The listing builds one solid part. Answer for the finished solid, in the listing's coordinates (mm). Face numbers are marked on the shaded views. A direction names the side the tool comes from. Round coordinates to 2 decimals unless told otherwise and drop trailing zeros. Loops run counter-clockwise (first coordinate to the right, second up) from the corner with the lowest first, then second, coordinate; pieces in that order, holes last. Notation, with made-up numbers: (-34, 59.5) -> (-11, 59.5) arc R7 ccw to (-11, 69.5) -> close; hole circle Ø10 at (58, -13). An arc over 180 degrees is marked (long way). Use a Markdown table: item, result. Add a question column.
Q1. For a pull along X with two mould halves and no side action, classify the marked faces 1, 2 and 3 as released by +X, released by -X, zero draft, split by the parting line, or undercut.
Q2. Section D-D on x = -76.5 is taken. Give the vertices of the cut face in (y, z).
Q3. Which of the six approach directions +Z, -Z, +X, -X, +Y, -Y give full straight-line access (tool end or side, diameter ignored) to the marked faces 4 and 5?
Q4. Consider line 1 (Y direction, x = -97, z = 180); line 2 (X direction, y = 27.5, z = 146.5); line 3 (X direction, y = 5, z = 2). Determine where each line is inside the solid, lowest interval first.
Q5. Section A-A on x = -10.5 is taken. Give the vertices of the cut face in (y, z), then the cut area to 3 significant figures.
Q6. Given pin 1 Ø2 at (x, y) = (-96, 72.5) entering from +Z; pin 2 Ø1.5 at (x, z) = (52, 31) entering from +Y; pin 3 Ø9.5 at (x, z) = (-2, 89.5) entering from +Y; pin 4 Ø2.5 at (x, z) = (96, 98) entering from +Y, each flat-ended and moving along its own axis, determine where each tip first touches the part or whether it passes through.
Q7. Section C-C on y = 34 is taken. Give the vertices of the cut face in (x, z).
from build123d import *

# Parameters (mm, degrees)
BOSS_EXTRUDE1_DEPTH = 225
BOSS_EXTRUDE2_DEPTH = 10
SKETCH6_W           = 210
SKETCH6_H           = 200
BOSS_EXTRUDE3_DEPTH = 15
SKETCH5_R           = 2.1
CUT_EXTRUDE1_DEPTH  = 6
SKETCH10_W          = 210
SKETCH10_H          = 200
BOSS_EXTRUDE4_DEPTH = 40
SKETCH11_R          = 4.75
BOSS_EXTRUDE5_DEPTH = 5
BOSS_EXTRUDE5_TAPER = 5
SKETCH13_W          = 185
SKETCH13_H          = 10
BOSS_EXTRUDE6_DEPTH = 47.5
SKETCH14_W          = 185
SKETCH14_H          = 10
BOSS_EXTRUDE7_DEPTH = 47.5
SKETCH7_W           = 21
SKETCH7_H           = 10.25
CUT_EXTRUDE2_DEPTH  = 15
SKETCH15_R          = 2.1
CUT_EXTRUDE4_DEPTH  = 4.5
CUT_EXTRUDE5_DEPTH  = 185
SKETCH17_W          = 210
SKETCH17_H          = 40
BOSS_EXTRUDE8_DEPTH = 10


with BuildPart() as part:
    # Sketch2 → Boss-Extrude1 (new body)
    with BuildSketch(Plane(origin=(0, 0, 0), x_dir=(1, 0, 0), z_dir=(0, 1, 0))):
        Polygon((-90, 0), (90, 0), (90, -185), (105, -185), (105, 15), (-105, 15), (-105, -185), (-90, -185), align=None)
    extrude(amount=BOSS_EXTRUDE1_DEPTH)

    # Sketch3 → Boss-Extrude2 (add)
    with BuildSketch(Plane(origin=(0, 10, 0), x_dir=(1, 0, 0), z_dir=(0, 1, 0))):
        Polygon((-90, -185), (-22.5, -185), (-22.5, -10), (22.5, -10), (22.5, -185), (90, -185), (90, 0), (-90, 0), align=None)
    extrude(amount=BOSS_EXTRUDE2_DEPTH)

    # Sketch6 → Boss-Extrude3 (add)
    with BuildSketch(Plane.XZ):
        with Locations((0, 85)):
            Rectangle(SKETCH6_W, SKETCH6_H)
    extrude(amount=BOSS_EXTRUDE3_DEPTH)

    # Sketch5 → Cut-Extrude1 (cut)
    with BuildSketch(Plane.XY.offset(185)):
        with Locations((-97.5, 217.5)):
            Circle(SKETCH5_R)
        with Locations((97.5, 217.5)):
            Circle(SKETCH5_R)
        with Locations((-97.5, -7.5)):
            Circle(SKETCH5_R)
        with Locations((97.5, -7.5)):
            Circle(SKETCH5_R)
    extrude(amount=-CUT_EXTRUDE1_DEPTH, mode=Mode.SUBTRACT)

    # Sketch10 → Boss-Extrude4 (add)
    with BuildSketch(Plane.XZ.offset(15)):
        with Locations((0, 85)):
            Rectangle(SKETCH10_W, SKETCH10_H)
    extrude(amount=BOSS_EXTRUDE4_DEPTH)

    # Sketch11 → Boss-Extrude5 (add)
    with BuildSketch(Plane(origin=(0, 0, 0), x_dir=(1, 0, 0), z_dir=(0, 1, 0))):
        with Locations((0, -90)):
            Circle(SKETCH11_R)
    extrude(amount=BOSS_EXTRUDE5_DEPTH, taper=BOSS_EXTRUDE5_TAPER)

    # Sketch13 → Boss-Extrude6 (add)
    with BuildSketch(Plane.ZY.offset(-90)):
        with Locations((92.5, 5)):
            Rectangle(SKETCH13_W, SKETCH13_H)
    extrude(amount=BOSS_EXTRUDE6_DEPTH)

    # Sketch14 → Boss-Extrude7 (add)
    with BuildSketch(Plane(origin=(-90, 0, 0), x_dir=(0, 0, -1), z_dir=(1, 0, 0))):
        with Locations((-92.5, 5)):
            Rectangle(SKETCH14_W, SKETCH14_H)
    extrude(amount=BOSS_EXTRUDE7_DEPTH)

    # Sketch7 → Cut-Extrude2 (cut)
    with BuildSketch(Plane(origin=(0, 0, -15), x_dir=(-1, 0, 0), z_dir=(0, 0, -1))):
        with Locations((-32, 5.125)):
            Rectangle(SKETCH7_W, SKETCH7_H)
    extrude(amount=-CUT_EXTRUDE2_DEPTH, mode=Mode.SUBTRACT)

    # Sketch15 → Cut-Extrude4 (cut)
    with BuildSketch(Plane(origin=(0, 225, 0), x_dir=(1, 0, 0), z_dir=(0, 1, 0))):
        with Locations((0, 7.5)):
            Circle(SKETCH15_R)
        with Locations((-97.5, -90)):
            Circle(SKETCH15_R)
        with Locations((97.5, -90)):
            Circle(SKETCH15_R)
    extrude(amount=-CUT_EXTRUDE4_DEPTH, mode=Mode.SUBTRACT)

    # Split1
    split(bisect_by=Plane.ZX.offset(75), keep=Keep.BOTTOM)

    # Sketch16 → Cut-Extrude5 (cut)
    with BuildSketch(Plane.XY.offset(185)):
        Polygon((-99.25, 75), (-99.25, 70), (-101.75, 70), (-101.75, 67.5), (-93.25, 67.5), (-93.25, 70), (-95.75, 70), (-95.75, 75), align=None)
        Polygon((95.75, 70), (95.75, 75), (99.25, 75), (99.25, 70), (101.75, 70), (101.75, 67.5), (93.25, 67.5), (93.25, 70), align=None)
    extrude(amount=-CUT_EXTRUDE5_DEPTH, mode=Mode.SUBTRACT)

    # Sketch17 → Boss-Extrude8 (add)
    with BuildSketch(Plane.XY.offset(185)):
        with Locations((0, -35)):
            Rectangle(SKETCH17_W, SKETCH17_H)
    extrude(amount=BOSS_EXTRUDE8_DEPTH)


solid = part.part
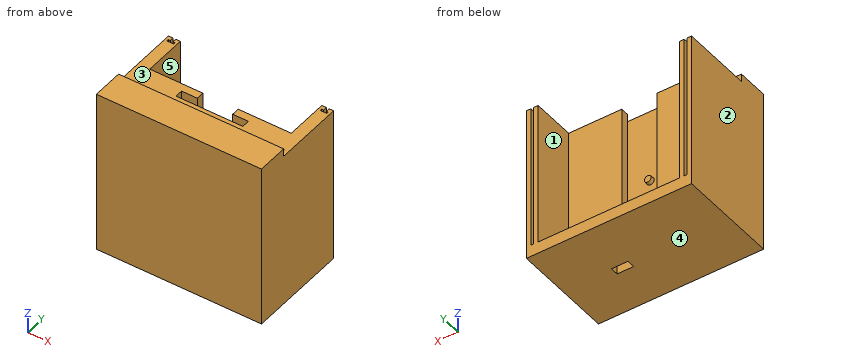
Checked values:
| question | item | result |
|---|---|---|
| 1 | face 1 | undercut |
| 1 | face 2 | released by -X |
| 1 | face 3 | zero draft |
| 2 | outline | (-55, -15) -> (75, -15) -> (75, 0) -> (20, 0) -> (20, 185) -> (-15, 185) -> (-15, 195) -> (-55, 195) -> close |
| 3 | face 4 | -Z, +X, -X, +Y, -Y |
| 3 | face 5 | +Z, +Y |
| 4 | line 1 | y = -55 to -9.54, -5.46 to 67.5 |
| 4 | line 2 | x = -105 to -90, 90 to 105 |
| 4 | line 3 | x = -105 to -42.5, 42.5 to 105 |
| 5 | outline | (-55, -15) -> (75, -15) -> (75, 0) -> (20, 0) -> (20, 10) -> (10, 10) -> (10, 0) -> (0, 0) -> (0, 185) -> (-15, 185) -> (-15, 195) -> (-55, 195) -> close |
| 5 | area | 12,600 mm2 |
| 6 | pin 1 | stops at z = 185 |
| 6 | pin 2 | stops at y = 20 |
| 6 | pin 3 | stops at y = 5 |
| 6 | pin 4 | stops at y = 75 |
| 7 | outline | (-105, -15) -> (105, -15) -> (105, 185) -> (90, 185) -> (90, 0) -> (-90, 0) -> (-90, 185) -> (-105, 185) -> close |
